Geometry: final body of the model. Coordinates: model frame, mm. Coordinates: 2 decimals unless noted, no trailing zeros. Loops run counter-clockwise (first coordinate to the right, second up) from the corner with the lowest first, then second, coordinate; pieces in that order, holes last. Notation, with made-up numbers: M -15.75,68 L 24.25,68 A21 cw 24.25,74 Z; hole C 7,-7.5 d4. An arc over 180 degrees is marked long. Write item = value, one per line. Start each with the question number.
```python
from build123d import *

# Parameters (mm, degrees)
F0_W     = 49.176914
F0_H     = 39.856406
F0_R     = 1
F1_DEPTH = 1.5
F2_R     = 1
F2_R_2   = 5
F3_DEPTH = 1.5


with BuildPart() as f1:
    # F0 (on Top) → F1 (new body)
    with BuildSketch(Plane.XY):
        Rectangle(F0_W, F0_H)
        with Locations((-11.588457, -15.928203)):
            Circle(F0_R, mode=Mode.SUBTRACT)
        with Locations((-19.588457, -2.071797)):
            Circle(F0_R, mode=Mode.SUBTRACT)
        with Locations((19.588457, 2.071797)):
            Circle(F0_R, mode=Mode.SUBTRACT)
        with Locations((11.588457, 15.928203)):
            Circle(F0_R, mode=Mode.SUBTRACT)
    extrude(amount=F1_DEPTH)

    # F2 (on face) → F3 (cut, through all)
    with BuildSketch(Plane.XY.offset(1.5)):
        with Locations((-10, 10)):
            Circle(F2_R)
        with Locations((10, 10)):
            Circle(F2_R)
        with Locations((-10, -10)):
            Circle(F2_R)
        with Locations((10, -10)):
            Circle(F2_R)
        Circle(F2_R_2)
    extrude(amount=-F3_DEPTH, mode=Mode.SUBTRACT)


solid = f1.part
```
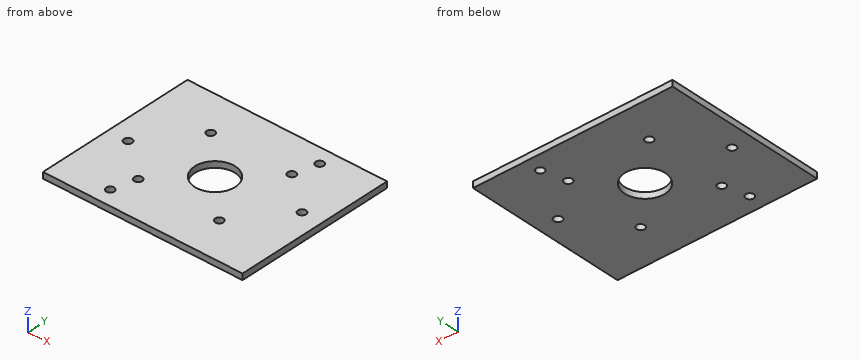
Item 1: Section query C-C (x = 0). Return the cut outline in (y, z).
Item 2: Line query: line 1 (Y direction, x = -10, z = 0.8); line 2 (X direction, y = -2.5, z = 0.6); line 3 (Y direction, x = -4, z = 1.1). Output: solid intervals per line, ascending. Write a range as from..to.
Item 3: Section query D-D (y = -4). Return the cut outline in (x, z), plus the area to 3 significant figures.
Item 4: Section query A-A (x = 10). Return the cut outline in (y, z), plus the area to 3 significant figures.
Item 5: Section query B-B (y = 10). Return the cut outline in (x, z).
Verdict:
q1.outline = M -19.93,0 L -5,0 L -5,1.5 L -19.93,1.5 Z; M 5,0 L 19.93,0 L 19.93,1.5 L 5,1.5 Z
q2.line_1 = -19.93..-11, -9..9, 11..19.93
q2.line_2 = -24.59..-20.49, -18.68..-4.33, 4.33..24.59
q2.line_3 = -19.93..-3, 3..19.93
q3.outline = M -24.59,0 L -3,0 L -3,1.5 L -24.59,1.5 Z; M 3,0 L 24.59,0 L 24.59,1.5 L 3,1.5 Z
q3.area = 64.8 mm2
q4.outline = M -19.93,0 L -11,0 L -11,1.5 L -19.93,1.5 Z; M -9,0 L 9,0 L 9,1.5 L -9,1.5 Z; M 11,0 L 19.93,0 L 19.93,1.5 L 11,1.5 Z
q4.area = 53.8 mm2
q5.outline = M -24.59,0 L -11,0 L -11,1.5 L -24.59,1.5 Z; M -9,0 L 9,0 L 9,1.5 L -9,1.5 Z; M 11,0 L 24.59,0 L 24.59,1.5 L 11,1.5 Z
